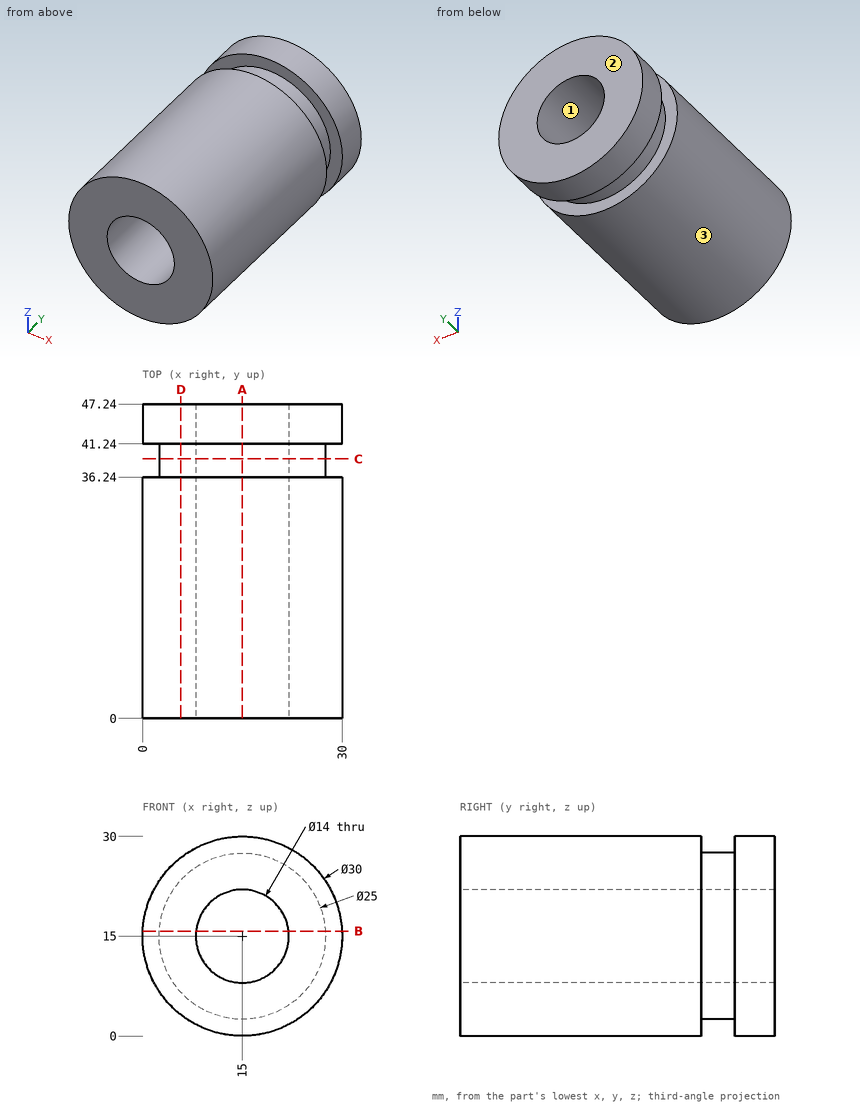
The drawing under review shows one solid part. Ordinate dimensions are in mm from its lowest x, y, z. Round coordinates to 2 decimals unless told otherwise and drop trailing zeros. Write each loop counter-clockwise with the first axis right and the second up, starting at its lowest first coordinate (ties: lowest second). Pieces come first, ordered by that corner, then holes. Notation, with made-up numbers: (51, -1.5) -> (82, -1.5) arc R13 cw to (82, 15.5) -> close; hole circle Ø7 at (82, -3.5). An arc over 180 degrees is marked (long way). Put each result on its own line as item: value.
Q1. The part is to be moulded in two halves that separate along X. For the marked faces 1, 2 and 3, say which applies: released by +X, released by -X, zero draft, split by the parting line, or undercut.
Determined:
face 1: undercut
face 2: zero draft
face 3: split by the parting line
Q2. Consider section C-C on y = 39. State the section outline as (x, z) points.
Determined:
outline: circle Ø25 at (15, 15); hole circle Ø14 at (15, 15)
Q3. Consider section B-B on z = 15.75. State the section outline as (x, y) points, and give its area (3 significant figures).
Determined:
outline: (0.02, 0) -> (8.04, 0) -> (8.04, 47.24) -> (0.02, 47.24) -> (0.02, 41.24) -> (2.52, 41.24) -> (2.52, 36.24) -> (0.02, 36.24) -> close; (21.96, 0) -> (29.98, 0) -> (29.98, 36.24) -> (27.48, 36.24) -> (27.48, 41.24) -> (29.98, 41.24) -> (29.98, 47.24) -> (21.96, 47.24) -> close
area: 733 mm^2
Q4. Consider section A-A on x = 15. State the section outline as (y, z) points, and give its area (3 significant figures).
Determined:
outline: (0, 0) -> (36.24, 0) -> (36.24, 2.5) -> (41.24, 2.5) -> (41.24, 0) -> (47.24, 0) -> (47.24, 8) -> (0, 8) -> close; (0, 22) -> (47.24, 22) -> (47.24, 30) -> (41.24, 30) -> (41.24, 27.5) -> (36.24, 27.5) -> (36.24, 30) -> (0, 30) -> close
area: 731 mm^2
Q5. To check wall thickness, follow L1, parallel to Y at x = 7.25, z = 4.75; L2, parallel to Z at x = 15, y = 19; L3, parallel to X at y = 13.5, z = 10. State the ranges of each line that lie inside material, in increasing order. Write a range as [from, to].
Determined:
L1: y = [0, 36.24], [41.24, 47.24]
L2: z = [0, 8], [22, 30]
L3: x = [0.86, 10.1], [19.9, 29.14]
Q6. Clearance check with flat-ended pins moving along their axes: pin 1 Ø6 at (x, z) = (8.5, 14) entering from -Y; pin 2 Ø6 at (y, z) = (28.5, 4.5) entering from -X; pin 3 Ø12 at (y, z) = (5, 24) entering from -X. State where each tip first meets the part, or that it passes through.
Determined:
pin 1: stops at y = 0
pin 2: stops at x = 2.01
pin 3: stops at x = 0.3
Q7. Consider section D-D on x = 5.75. State the section outline as (y, z) points, and give its area (3 significant figures).
Determined:
outline: (0, 3.19) -> (36.24, 3.19) -> (36.24, 6.59) -> (41.24, 6.59) -> (41.24, 3.19) -> (47.24, 3.19) -> (47.24, 26.81) -> (41.24, 26.81) -> (41.24, 23.41) -> (36.24, 23.41) -> (36.24, 26.81) -> (0, 26.81) -> close
area: 1,080 mm^2
